Here's how the part is built. I have some questions about the finished solid (model axes, mm). Face numbers are marked on the shaded views. A direction names the side the tool comes from. Round coordinates to 2 decimals unless told otherwise and drop trailing zeros. Order: outer loops, then holes, each group sorted by start corner. A loop starts at its lowest first (then second) coordinate and runs counter-clockwise, first axis right, second up.
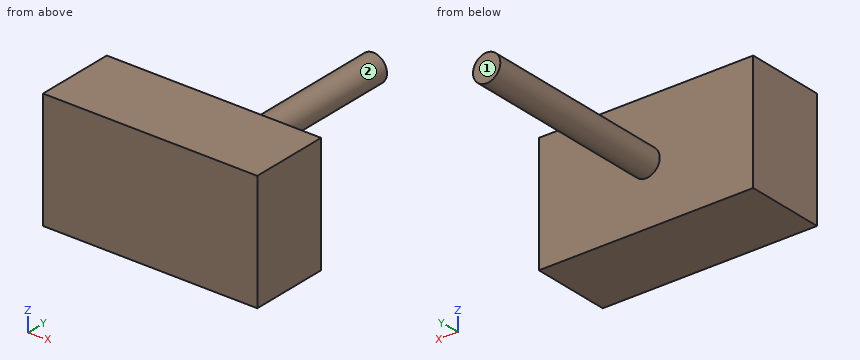
```python
from build123d import *

# Parameters (mm, degrees)
F0_R     = 17.4638157323
F1_DEPTH = 254
F3_DEPTH = 76.2
F4_DEPTH = 25.4


with BuildPart() as f1:
    # F0 (on Front) → F1 (new body)
    with BuildSketch(Plane.XZ):
        Circle(F0_R)
    extrude(amount=F1_DEPTH)

    # F2 (on face) → F3 (join)
    with BuildSketch(Plane.XZ.offset(254)):
        with BuildLine():
            Line((-17.4638157323, 0), (0, 0))
            Line((0, 0), (0, 17.4638157323))
            ThreePointArc((0, 17.4638157323), (-12.3487825297, 12.3487825297), (-17.4638157323, 0))
        make_face()
        with BuildLine():
            Line((0, -17.4638157323), (0, 0))
            Line((0, 0), (-17.4638157323, 0))
            ThreePointArc((-17.4638157323, 0), (-12.3487825297, -12.3487825297), (0, -17.4638157323))
        make_face()
        with BuildLine():
            ThreePointArc((0, -17.4638157323), (-12.3487825297, -12.3487825297), (-17.4638157323, 0))
            Line((-17.4638157323, 0), (-137.0784789324, 0))
            Line((-137.0784789324, 0), (-137.0784789324, -75.2277523279))
            Line((-137.0784789324, -75.2277523279), (0, -75.2277523279))
            Line((0, -75.2277523279), (0, -17.4638157323))
        make_face()
        with BuildLine():
            Line((0, 17.4638157323), (0, 0))
            Line((0, 0), (17.4638157323, 0))
            ThreePointArc((17.4638157323, 0), (12.3487825297, 12.3487825297), (0, 17.4638157323))
        make_face()
        with BuildLine():
            Line((0, 75.2277523279), (0, 17.4638157323))
            ThreePointArc((0, 17.4638157323), (12.3487825297, 12.3487825297), (17.4638157323, 0))
            Line((17.4638157323, 0), (137.0784789324, 0))
            Line((137.0784789324, 0), (137.0784789324, 75.2277523279))
            Line((137.0784789324, 75.2277523279), (0, 75.2277523279))
        make_face()
        with BuildLine():
            Line((137.0784789324, 0), (17.4638157323, 0))
            ThreePointArc((17.4638157323, 0), (12.3487825297, -12.3487825297), (0, -17.4638157323))
            Line((0, -17.4638157323), (0, -75.2277523279))
            Line((0, -75.2277523279), (137.0784789324, -75.2277523279))
            Line((137.0784789324, -75.2277523279), (137.0784789324, 0))
        make_face()
        with BuildLine():
            Line((17.4638157323, 0), (0, 0))
            Line((0, 0), (0, -17.4638157323))
            ThreePointArc((0, -17.4638157323), (12.3487825297, -12.3487825297), (17.4638157323, 0))
        make_face()
        with BuildLine():
            Line((-137.0784789324, 0), (-17.4638157323, 0))
            ThreePointArc((-17.4638157323, 0), (-12.3487825297, 12.3487825297), (0, 17.4638157323))
            Line((0, 17.4638157323), (0, 75.2277523279))
            Line((0, 75.2277523279), (-137.0784789324, 75.2277523279))
            Line((-137.0784789324, 75.2277523279), (-137.0784789324, 0))
        make_face()
    extrude(amount=F3_DEPTH)

    # F4 (add): a face of the model
    f4_faces = [f1.faces().sort_by_distance(p)[0] for p in [
        (0, -330.2, 0),
    ]]
    extrude(f4_faces, amount=F4_DEPTH)


solid = f1.part
```
1. If we section it at C-C, the plane y = -178: Write out the boundary of the cut face in (x, z).
Evaluation:
outline: circle Ø34.93 at (0, 0)
2. I need wall thicknesses on probe 1 along Y at (x, z) = (120, -35.5); probe 2 along X at (y, z) = (-218.5, 14); probe 3 along X at (y, z) = (-14.5, -9.5). Which ranges of each line are inside material? Lowest first, please.
Evaluation:
probe 1: y = -355.6 to -254
probe 2: x = -10.44 to 10.44
probe 3: x = -14.65 to 14.65
3. If we section it at A-A, the plane x = 0: Write out the boundary of the cut face in (y, z).
Evaluation:
outline: (-355.6, -75.23) - (-254, -75.23) - (-254, -17.46) - (0, -17.46) - (0, 17.46) - (-254, 17.46) - (-254, 75.23) - (-355.6, 75.23) - close
4. If we section it at D-D, the plane z = -39: Write out the boundary of the cut face in (x, y), and give its area (3 significant figures).
Evaluation:
outline: (-137.08, -355.6) - (137.08, -355.6) - (137.08, -254) - (-137.08, -254) - close
area: 27,900 mm2
5. I'm going to push flat-ended pins straight in: P1, Ø2, axis at y = -170, z = 2, coming from the -X side; P2, Ø4, axis at x = 35, z = -6.5, coming from the +Y side; P3, Ø5, axis at x = 7.5, y = -162.5, coming from the -Z side. Where does each tip first touch, or does it pass through?
Evaluation:
P1: stops at x = -17.44
P2: stops at y = -254
P3: stops at z = -16.73
6. On a 3-axis mill with a long thin cutter (end or side, diameter ignored), from which of +Z, -Z, +X, -X, +Y, -Y can I reach the whole of each face in a straight line? I mean the marked faces 1 and 2. Say none if no direction works.
Evaluation:
face 1: +Z, -Z, +X, -X, +Y
face 2: +Y
7. If we section it at B-B, the plane z = 0: Write out the boundary of the cut face in (x, y), and give its area (3 significant figures).
Evaluation:
outline: (-137.08, -355.6) - (137.08, -355.6) - (137.08, -254) - (17.46, -254) - (17.46, 0) - (-17.46, 0) - (-17.46, -254) - (-137.08, -254) - close
area: 36,700 mm2
